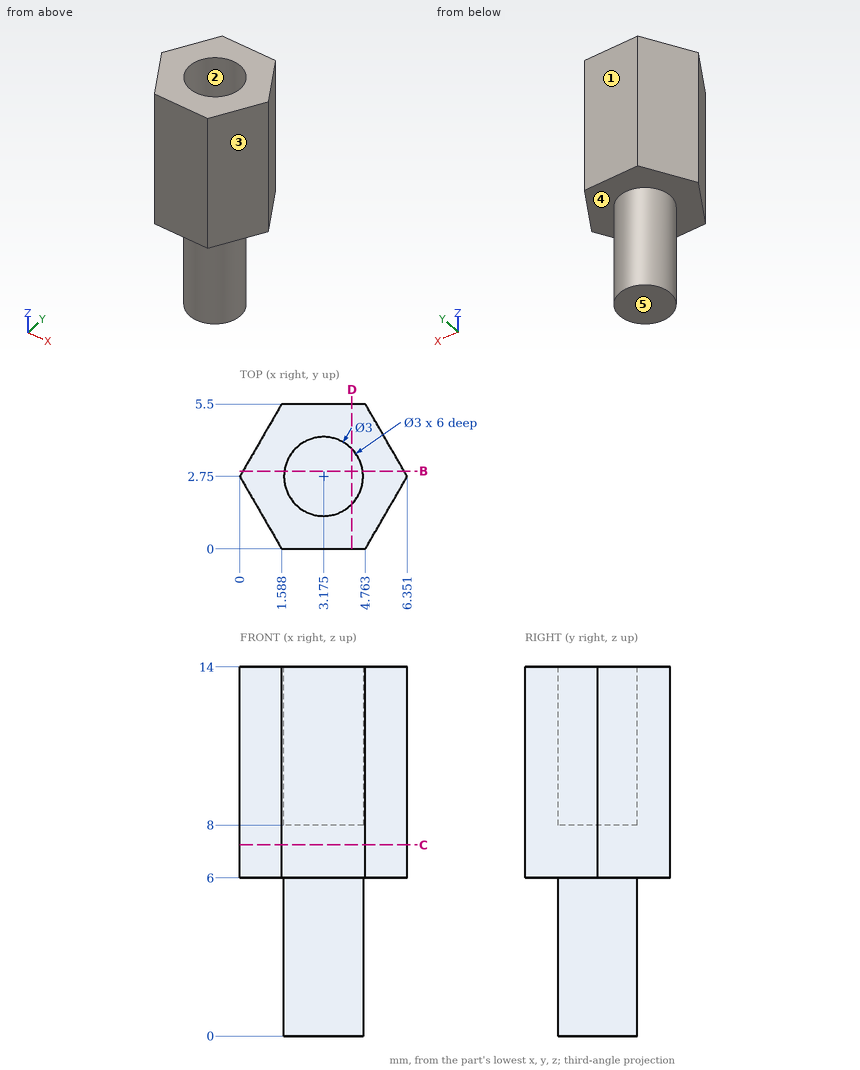
Job drawing, mm, ordinate dimensions from the low corner. One solid piece. A direction names the side the tool comes from. Coordinates: 2 decimals unless noted, no trailing zeros. Write each loop counter-clockwise with the first axis right and the second up, starting at its lowest first coordinate (ties: lowest second). Pieces come first, ordered by that corner, then holes.
Item 1: Slice it at C-C (z = 7.25). Write the cut outline in (x, y).
Item 2: Which spindle directions (+Z, -Z, +X, -X, +Y, -Y) get a long thin tool onto all of the face, cutting with end or side? Do the marked faces 4 and 5. Say none if no direction does.
Item 3: Pin check, flat tips, straight feed: pin 1 (1 mm diameter, centred on y = 1, z = 3.5, fed in from +X) (1 decimal); pin 2 (2 mm diameter, centred on y = 4.5, z = 8, fed in from -X). Stop position of each tip, or through.
Item 4: Probe line 1 (Z direction, x = 2.5, y = 2.65); line 2 (Z direction, x = 5.5, y = 1.8); line 3 (Y direction, x = 2.5, z = 13). List the from-to ranges inside material, lowest first.
Item 5: Slice it at D-D (x = 4.25). Write the cut outline in (y, z).
Item 6: Slice it at B-B (y = 2.95). Write the cut outline in (x, z) (1 decimal).
Item 7: Mould opens along Y. For the marked faces 1, 2 and 3 say: released by +Y, released by -Y, zero draft, split by the parting line, or undercut.
Results found:
1. outline: (0, 2.75) - (1.59, 0) - (4.76, 0) - (6.35, 2.75) - (4.76, 5.5) - (1.59, 5.5) - close
2. face 4: -Z
2. face 5: -Z, +X, -X, +Y, -Y
3. pin 1: stops at x = 4
3. pin 2: stops at x = 0.43
4. line 1: z = 0 to 8
4. line 2: z = 6 to 14
4. line 3: y = 0 to 1.41, 4.09 to 5.5
5. outline: (0, 6) - (1.7, 6) - (1.7, 0) - (3.8, 0) - (3.8, 6) - (5.5, 6) - (5.5, 14) - (3.8, 14) - (3.8, 8) - (1.7, 8) - (1.7, 14) - (0, 14) - close
6. outline: (0.1, 6) - (1.7, 6) - (1.7, 0) - (4.7, 0) - (4.7, 6) - (6.2, 6) - (6.2, 14) - (4.7, 14) - (4.7, 8) - (1.7, 8) - (1.7, 14) - (0.1, 14) - close
7. face 1: released by +Y
7. face 2: undercut
7. face 3: released by -Y
